Part print with two shaded views. Sizes in mm from the minimum x, y, z corner. A direction names the side the tool comes from. Give positions to 0.01 mm unless a question says otherwise; leave off trailing zeros. Loops run counter-clockwise (first coordinate to the right, second up) from the corner with the lowest first, then second, coordinate; pieces in that order, holes last. Notation, with made-up numbers: M 37.25,-1 L 44.25,-1 A18 cw 44.25,9 Z; hole C -16.5,-7.5 d3. An arc over 180 degrees is marked long. Answer as a JSON object with one key per item and string values. Group by question number.
1. Slice it at B-B (z = 16). List the corners of the cut face in (x, y).
2. Drill centre lines: line 1 along Y through (x, z) = (25.5, 33); line 2 along X through (y, z) = (53, 14.5); line 3 along Z through (x, y) = (17.5, 45). Where is each one in solid material? Low to high. Write a range as [from, to].
3. Mould opens along X. For the marked faces 3, 4 and 5 say: released by +X, released by -X, zero draft, split by the parting line, or undercut.
4. Slice it at D-D (y = 55). List the corners of the cut face in (x, z), then the cut area to 3 significant figures.
5. Drop flat-ended pins along their axis: pin 1 Ø5 at (x, z) = (66.5, 5) entering from -Y; pin 2 Ø5 at (x, y) = (5, 7) entering from +Z; pin 3 Ø1.3 at (x, y) = (5, 7) entering from -Z; pin 4 Ø1 at (y, z) = (31, 24) entering from -X. Give the stop position or say it passes through.
6. Slice it at A-A (z = 32). List the corners of the cut face in (x, y).
7. Slice it at C-C (x = 5). List the corners of the cut face in (y, z), then the cut area to 3 significant figures.
8. 3-axis set-ups, long thin cutter, end or side, ignore diameter. For the marked faces 1 and 2: which of +Z, -Z, +X, -X, +Y, -Y reach the whole face in a straight line?
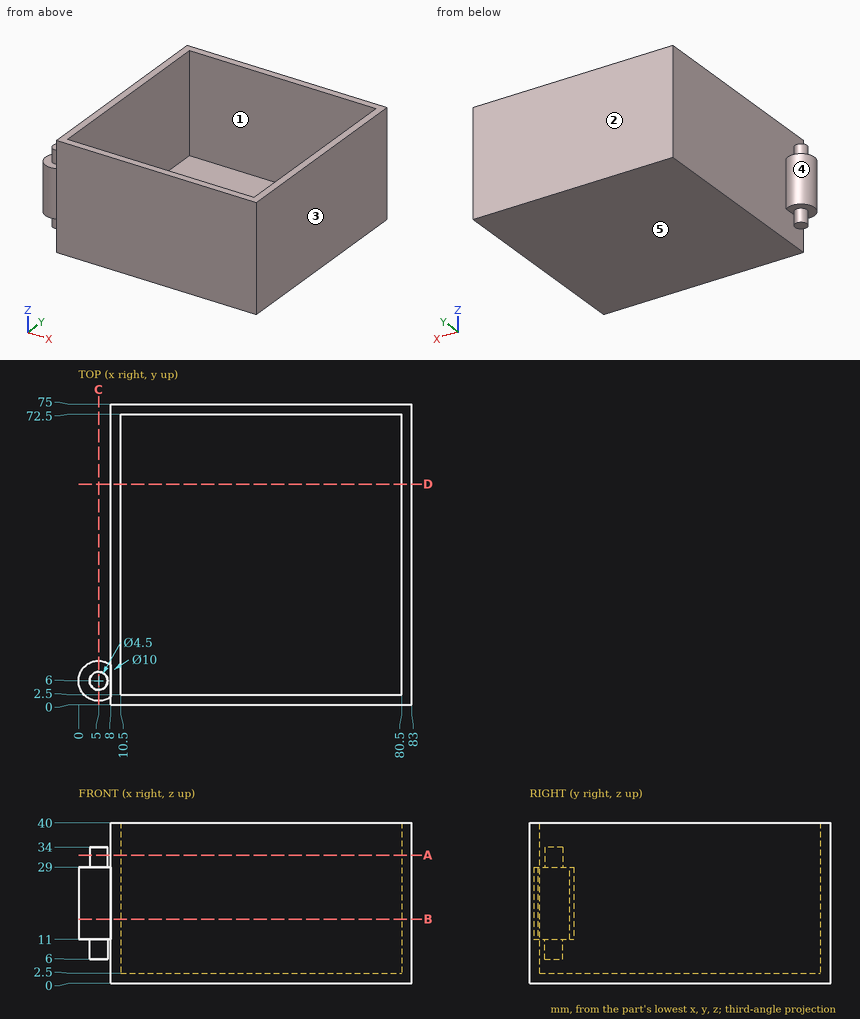
Established:
{
 "1": {"outline": "M 8,0 L 83,0 L 83,75 L 8,75 L 8,10 A5 ccw long 8,2 Z; hole M 10.5,2.5 L 80.5,2.5 L 80.5,72.5 L 10.5,72.5 Z"},
 "2": {"line 1": "y = [0, 2.5], [72.5, 75]", "line 2": "x = [8, 10.5], [80.5, 83]", "line 3": "z = [0, 2.5]"},
 "3": {"face 3": "released by +X", "face 4": "undercut", "face 5": "zero draft"},
 "4": {"outline": "M 8,0 L 83,0 L 83,40 L 80.5,40 L 80.5,2.5 L 10.5,2.5 L 10.5,40 L 8,40 Z", "area": "375 mm^2"},
 "5": {"pin 1": "stops at y = 0", "pin 2": "stops at z = 34", "pin 3": "stops at z = 6", "pin 4": "stops at x = 8"},
 "6": {"outline": "C 5,6 d4.5; M 8,0 L 83,0 L 83,75 L 8,75 Z; hole M 10.5,2.5 L 80.5,2.5 L 80.5,72.5 L 10.5,72.5 Z"},
 "7": {"outline": "M 1,11 L 3.75,11 L 3.75,6 L 8.25,6 L 8.25,11 L 11,11 L 11,29 L 8.25,29 L 8.25,34 L 3.75,34 L 3.75,29 L 1,29 Z", "area": "225 mm^2"},
 "8": {"face 1": "+Z", "face 2": "+Z, -Z, +X, -X, +Y"}
}
